The drawing under review shows one solid part. Ordinate dimensions are in mm from its lowest x, y, z. Coordinates: 2 decimals unless noted, no trailing zeros. Order: outer loops, then holes, each group sorted by start corner. A loop starts at its lowest first (then second) coordinate and runs counter-clockwise, first axis right, second up.
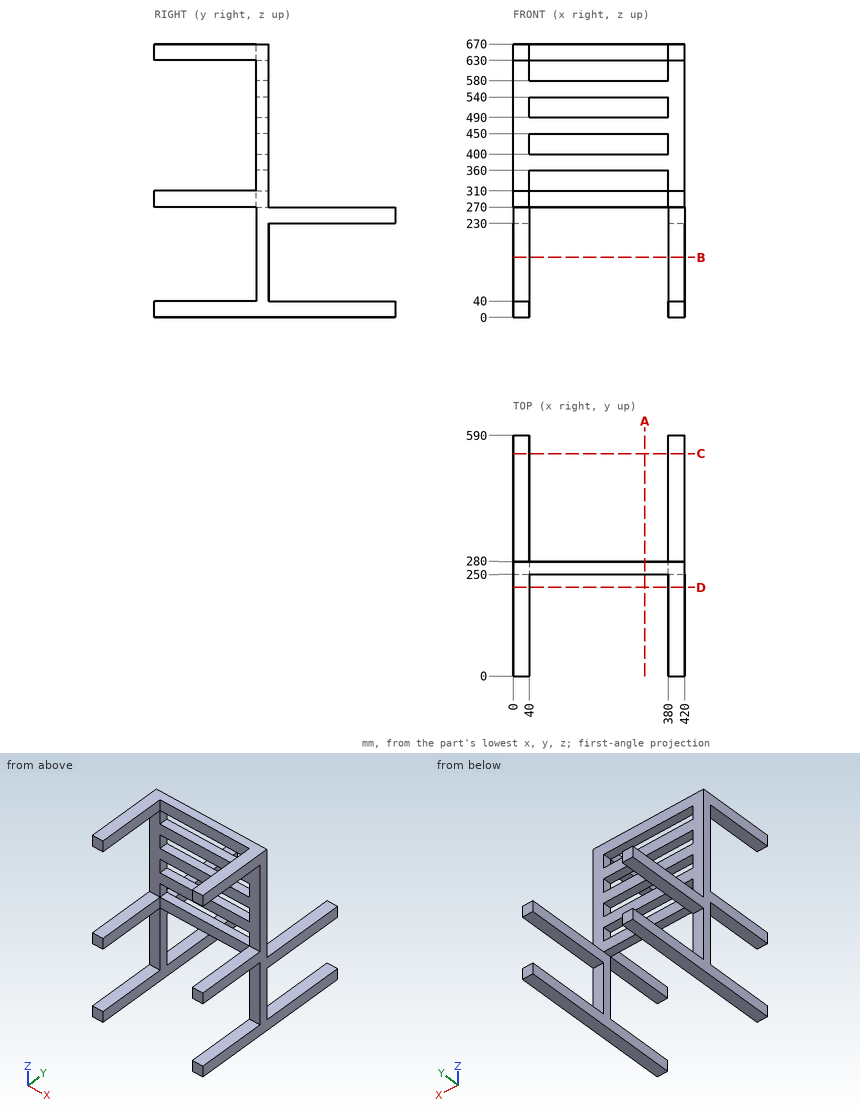
1. Clearance check with flat-ended pins moving along their axes: pin 1 Ø3 at (x, z) = (106.5, 281.5) entering from -Y; pin 2 Ø20 at (x, y) = (27.5, 395) entering from +Z; pin 3 Ø12 at (x, z) = (18.5, 172.5) entering from +Y. State where each tip first meets the part, or that it passes through.
Answer below:
pin 1: stops at y = 250
pin 2: stops at z = 270
pin 3: stops at y = 280
2. To check wall thickness, follow L1, parallel to Z at x = 345.5, y = 257.5; L2, parallel to Y at x = 396, z = 215.5. State the ranges of each line that lie inside material, in increasing order.
Answer below:
L1: z = 270 to 310, 360 to 400, 450 to 490, 540 to 580, 630 to 670
L2: y = 250 to 280
3. Take a section at D-D, the plane y = 217.5. Give the boundary of the cut face in (x, z).
Answer below:
outline: (0, 0) - (40, 0) - (40, 40) - (0, 40) - close; (0, 270) - (40, 270) - (40, 310) - (0, 310) - close; (0, 630) - (40, 630) - (40, 670) - (0, 670) - close; (380, 0) - (420, 0) - (420, 40) - (380, 40) - close; (380, 270) - (420, 270) - (420, 310) - (380, 310) - close; (380, 630) - (420, 630) - (420, 670) - (380, 670) - close
4. Take a section at C-C, the plane y = 545. Give the boundary of the cut face in (x, z), plus the area to 3 significant figures.
Answer below:
outline: (0, 0) - (40, 0) - (40, 40) - (0, 40) - close; (0, 230) - (40, 230) - (40, 270) - (0, 270) - close; (380, 0) - (420, 0) - (420, 40) - (380, 40) - close; (380, 230) - (420, 230) - (420, 270) - (380, 270) - close
area: 6,400 mm2
5. Take a section at B-B, the plane z = 147. Give the boundary of the cut face in (x, y), plus the area to 3 significant figures.
Answer below:
outline: (0, 250) - (40, 250) - (40, 280) - (0, 280) - close; (380, 250) - (420, 250) - (420, 280) - (380, 280) - close
area: 2,400 mm2
6. Take a section at A-A, the plane x = 323. Give the boundary of the cut face in (y, z), plus the area to 3 significant figures.
Answer below:
outline: (250, 270) - (280, 270) - (280, 310) - (250, 310) - close; (250, 360) - (280, 360) - (280, 400) - (250, 400) - close; (250, 450) - (280, 450) - (280, 490) - (250, 490) - close; (250, 540) - (280, 540) - (280, 580) - (250, 580) - close; (250, 630) - (280, 630) - (280, 670) - (250, 670) - close
area: 6,000 mm2
